For this review, take the finished solid that the model builds, in its own axes (mm). A direction names the side the tool comes from. Round coordinates to 2 decimals unless told otherwise and drop trailing zeros. Loops run counter-clockwise (first coordinate to the right, second up) from the corner with the lowest first, then second, coordinate; pieces in that order, holes last.
1) Mouldability with a two-part tool opening along Y and no side actions: class faces 4 (the flat face through (51.454, 28, 14)), 5 (the flat face through (-8, 100, 12)), 6 (the flat face through (-23.046, 57, 12)) as pulls with the +Y half, pulls with the -Y half, needs draft (parallel to the pull), parting line crosses it, or undercut.
2) Take a section at C-C (y = 51). State the section outline as (x, z) points, then the cut area to 3 significant figures.
3) Insertion check: pin 1 (1.4 mm diameter, centred on x = -3.28, y = 14.57, fed in from +Z); pin 2 (13.5 mm diameter, centred on x = 77, z = 20, fed in from +Y) (3 decimals). Each pin has a flat end and moves straight along its axis. Give the tip position at first contact, or say it passes through.
4) Take a section at B-B (x = 62). State the section outline as (y, z) points (3 decimals).
5) Wall thickness on L1, parallel to X at y = 57.5, z = 18; L2, parallel to X at y = 28, z = 24.75; L3, parallel to X at y = 18, z = 16.25: over which ranges is each line inside the solid? List them lowest first.
6) Take a section at D-D (z = 8.5). Give the number of separate pieces and of enclosed holes in the cut face, then the cut area to 3 significant figures.
7) Take a section at A-A (y = 79.5). State the section outline as (x, z) points.
8) Tool access review of faces 1 (the flat face through (102, 100, 12)), 2 (the flat face through (6.954, 70, 12)), 3 (the flat face through (1.975, 41, 14)): name each direction out of +Z, -Z, +X, -X, +Y, -Y from which nothing blocks a thin tool from reaching the whole face with its end or side.
```python
from build123d import *

# Parameters (mm, degrees)
BOSS_EXTRUDE1_DEPTH = 26.8
SKETCH2_W           = 20.5
SKETCH2_H           = 43.5
SKETCH2_W_2         = 43.5
SKETCH2_H_2         = 20.5
CUT_EXTRUDE1_DEPTH  = 157.194070808
SKETCH3_R           = 1.15
BOSS_EXTRUDE2_DEPTH = 26.8
SKETCH3_2_R         = 1.15
CUT_EXTRUDE2_DEPTH  = 157.194070808
SKETCH4_R           = 1.15
CUT_EXTRUDE3_DEPTH  = 157.194070808
FILLET1_R           = 2.3


with BuildPart() as part:
    # Sketch1 → Boss-Extrude1 (new body)
    with BuildSketch(Plane.XY):
        Polygon((86.954468728, 12.865007186), (116.954468728, 12.865007186), (116.954468728, 100), (86.954468728, 100), (86.954468728, 42.865007186), (6.954468728, 42.865007186), (6.954468728, 100), (-23.045531272, 100), (-23.045531272, 12.865007186), (6.954468728, 12.865007186), align=None)
    extrude(amount=BOSS_EXTRUDE1_DEPTH)

    # Sketch2 → Cut-Extrude1 (cut, through all)
    with BuildSketch(Plane.XY.offset(26.8)):
        with Locations((-8.275140501, 41.615007186)):
            Rectangle(SKETCH2_W, SKETCH2_H)
        with Locations((73.204468728, 27.895224973)):
            Rectangle(SKETCH2_W_2, SKETCH2_H_2)
    extrude(amount=-CUT_EXTRUDE1_DEPTH, mode=Mode.SUBTRACT)

    # Sketch3 → Boss-Extrude2 (add, through all)
    with BuildSketch(Plane.XY.offset(26.8)):
        with Locations((-13.275140501, 14.565007186)):
            Circle(SKETCH3_R)
        with Locations((-3.275140501, 14.565007186)):
            Circle(SKETCH3_R)
        with Locations((-13.275140501, 65.665007186)):
            Circle(SKETCH3_R)
        with Locations((-3.275140501, 65.665007186)):
            Circle(SKETCH3_R)
    extrude(amount=-BOSS_EXTRUDE2_DEPTH)

    # Sketch3<2> → Cut-Extrude2 (cut, through all)
    with BuildSketch(Plane.XY.offset(26.8)):
        with Locations((-13.275140501, 14.565007186)):
            Circle(SKETCH3_2_R)
        with Locations((-3.275140501, 14.565007186)):
            Circle(SKETCH3_2_R)
        with Locations((-13.275140501, 65.665007186)):
            Circle(SKETCH3_2_R)
        with Locations(Location((-3.275140501, 65.665007186, 0), (0, 0, 180))):
            Circle(SKETCH3_2_R)
    extrude(amount=-CUT_EXTRUDE2_DEPTH, mode=Mode.SUBTRACT)

    # Sketch4 → Cut-Extrude3 (cut, through all)
    with BuildSketch(Plane.XY.offset(26.8)):
        with Locations((100.254468728, 22.895224973)):
            Circle(SKETCH4_R)
        with Locations(Location((100.254468728, 32.895224973, 0), (0, 0, 180))):
            Circle(SKETCH4_R)
        with Locations((49.154468728, 22.895224973)):
            Circle(SKETCH4_R)
        with Locations(Location((49.154468728, 32.895224973, 0), (0, 0, 180))):
            Circle(SKETCH4_R)
    extrude(amount=-CUT_EXTRUDE3_DEPTH, mode=Mode.SUBTRACT)

    # Fillet1
    fillet1_edges = [part.edges().sort_by_distance(p)[0] for p in [
        (6.954468728, 100, 13.4),
        (86.954468728, 100, 13.4),
        (116.954468728, 100, 13.4),
        (116.954468728, 12.865007186, 13.4),
        (-23.045531272, 12.865007186, 13.4),
        (-23.045531272, 100, 13.4),
        (116.954468728, 56.432503593, 26.8),
        (101.954468728, 100, 26.8),
        (86.954468728, 71.432503593, 26.8),
        (46.954468728, 42.865007186, 26.8),
        (6.954468728, 71.432503593, 26.8),
        (-8.045531272, 100, 26.8),
        (-23.045531272, 56.432503593, 26.8),
    ]]
    fillet(fillet1_edges, radius=FILLET1_R)


solid = part.part
```
Response:
1. face 4: undercut
1. face 5: pulls with the +Y half
1. face 6: needs draft
2. outline: (-23.05, 0) - (-18.53, 0) - (-18.53, 26.8) - (-20.75, 26.8) arc R2.3 ccw to (-23.05, 24.5) - close; (1.97, 0) - (6.95, 0) - (6.95, 24.5) arc R2.3 ccw to (4.65, 26.8) - (1.97, 26.8) - close; (86.95, 0) - (116.95, 0) - (116.95, 24.5) arc R2.3 ccw to (114.65, 26.8) - (89.25, 26.8) arc R2.3 ccw to (86.95, 24.5) - close
2. area: 1,050 mm2
3. pin 1: passes through
3. pin 2: stops at y = 42.865
4. outline: (12.865, 0) - (17.645, 0) - (17.645, 26.8) - (12.865, 26.8) - close; (38.145, 0) - (42.865, 0) - (42.865, 24.5) arc R2.3 ccw to (40.565, 26.8) - (38.145, 26.8) - close
5. L1: x = -23.05 to -18.53, 1.97 to 6.95, 86.95 to 116.95
5. L2: x = -23.03 to -18.53, 1.97 to 51.45, 94.95 to 116.94
5. L3: x = -23.05 to 51.45, 94.95 to 116.95
6. separate pieces: 1
6. enclosed holes: 10
6. area: 5,800 mm2
7. outline: (-23.05, 0) - (6.95, 0) - (6.95, 24.5) arc R2.3 ccw to (4.65, 26.8) - (-20.75, 26.8) arc R2.3 ccw to (-23.05, 24.5) - close; (86.95, 0) - (116.95, 0) - (116.95, 24.5) arc R2.3 ccw to (114.65, 26.8) - (89.25, 26.8) arc R2.3 ccw to (86.95, 24.5) - close
8. face 1: +Z, -Z, +X, -X, +Y
8. face 2: +Z, -Z, +Y
8. face 3: +Z, -Z
